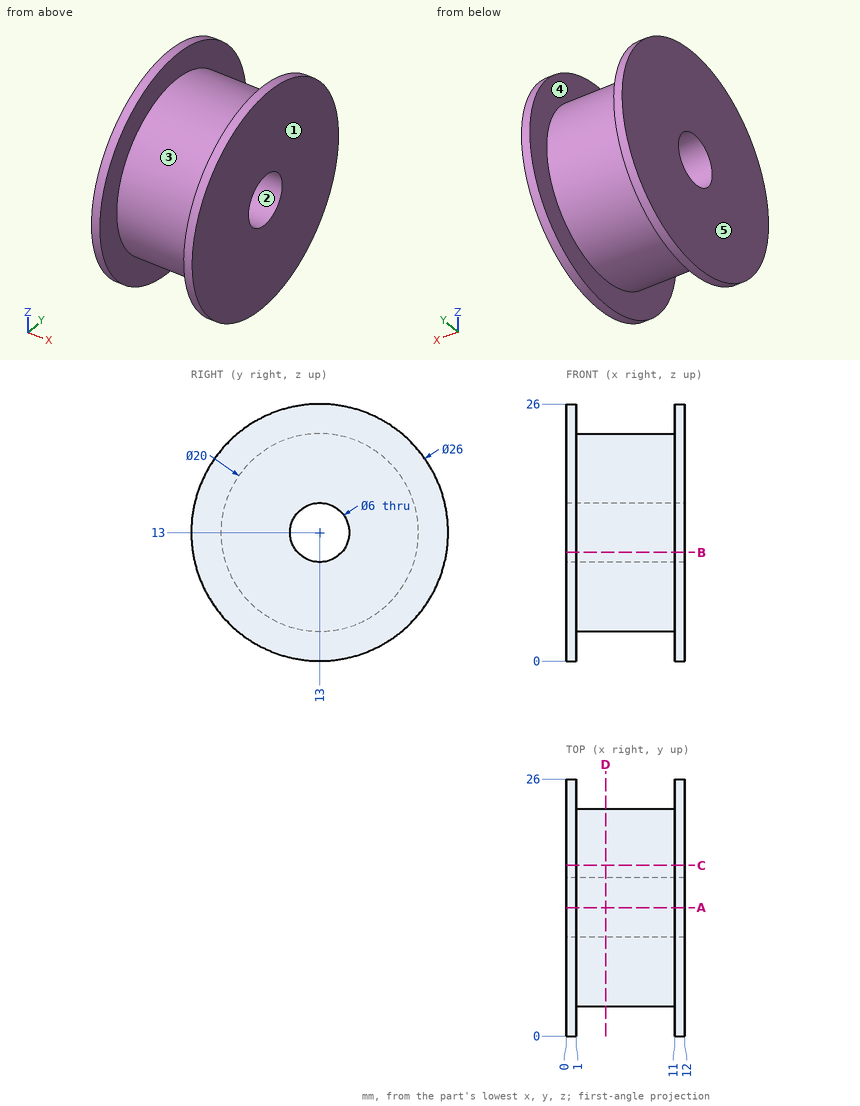
Here's the drawing with two shaded views (mm, measured from the low corner). I have some questions. A direction names the side the tool comes from. Round coordinates to 2 decimals unless told otherwise and drop trailing zeros. Loops run counter-clockwise (first coordinate to the right, second up) from the corner with the lowest first, then second, coordinate; pieces in that order, holes last. Notation, with made-up numbers: (31, -22.5) - (36, -22.5) arc R17 cw to (36, 7.5) - close; hole circle Ø8 at (30, 77.25). An arc over 180 degrees is marked (long way). Use CSV: the item, a comma, the result in double quotes. Start each with the question number.
1) If we section it at D-D on x = 4: Write out the boundary of the cut face in (y, z), plus the area to 3 significant figures.
2) For the marked faces 4 and 5, which set-ups out of +Z, -Z, +X, -X, +Y, -Y let a thin tool reach every point of the face, with its end or its side?
3) We'd pull the mould along Y, two halves only. Please class the marked faces 1, 2 and 3: released by +Y, released by -Y, zero draft, split by the parting line, or undercut.
4) Please list where these lines run through material, in increasing order: probe 1 along X at (y, z) = (5.5, 20.25); probe 2 along Y at (x, z) = (7.75, 13); probe 3 along Z at (x, y) = (9, 11.75). Write a range as [from, to].
5) If we section it at B-B on z = 11: Write out the boundary of the cut face in (x, y).
6) If we section it at A-A on y = 13: Write out the boundary of the cut face in (x, z).
7) If we section it at C-C on y = 17.25: Write out the boundary of the cut face in (x, z), plus the area to 3 significant figures.
8) For pin 1 Ø5 at (x, y) = (4, 15) entering from +Z; pin 2 Ø6 at (x, z) = (10, 6.5) entering from -Y; pin 3 Ø6 at (x, z) = (10, 20) entering from -Y; pin 4 Ø5 at (y, z) = (13, 13) entering from -X, each with a flat end and sliding along its axis, tell me the tip position at first contact or that it passes through.
Geometry results:
1,outline,"circle Ø20 at (13, 13); hole circle Ø6 at (13, 13)"
1,area,"286 mm2"
2,face 4,"none"
2,face 5,"+Z, -Z, -X, +Y, -Y"
3,face 1,"zero draft"
3,face 2,"undercut"
3,face 3,"split by the parting line"
4,probe 1,"x = [0, 1], [11, 12]"
4,probe 2,"y = [3, 10], [16, 23]"
4,probe 3,"z = [3.08, 10.27], [15.73, 22.92]"
5,outline,"(0, 0.15) - (1, 0.15) - (1, 3.2) - (11, 3.2) - (11, 0.15) - (12, 0.15) - (12, 10.76) - (0, 10.76) - close; (0, 15.24) - (12, 15.24) - (12, 25.85) - (11, 25.85) - (11, 22.8) - (1, 22.8) - (1, 25.85) - (0, 25.85) - close"
6,outline,"(0, 0) - (1, 0) - (1, 3) - (11, 3) - (11, 0) - (12, 0) - (12, 10) - (0, 10) - close; (0, 16) - (12, 16) - (12, 26) - (11, 26) - (11, 23) - (1, 23) - (1, 26) - (0, 26) - close"
7,outline,"(0, 0.71) - (1, 0.71) - (1, 3.95) - (11, 3.95) - (11, 0.71) - (12, 0.71) - (12, 25.29) - (11, 25.29) - (11, 22.05) - (1, 22.05) - (1, 25.29) - (0, 25.29) - close"
7,area,"230 mm2"
8,pin 1,"stops at z = 23"
8,pin 2,"stops at y = 0.53"
8,pin 3,"stops at y = 0.69"
8,pin 4,"passes through"
